```python
from build123d import *

# Parameters (mm, degrees)
BOSS_EXTRUDE1_DEPTH = 6
SKETCH3_R           = 3.5
SKETCH3_R_2         = 7
CUT_EXTRUDE1_DEPTH  = 83.160412203
FILLET1_R           = 2


with BuildPart() as part:
    # Sketch1 → Revolve1 (revolve)
    with BuildSketch(Plane(origin=(0, 0, 0), x_dir=(0, 0, -1), z_dir=(1, 0, 0)), mode=Mode.PRIVATE) as revolve1_sk:
        with BuildLine():
            Line((-3, 45), (-3, 26))
            ThreePointArc((-3, 26), (-3.878679656, 23.878679656), (-6, 23))
            Line((-6, 23), (-7, 23))
            Line((-7, 23), (-7, 7))
            Line((-7, 7), (0, 7))
            Line((0, 7), (0, 19))
            Line((0, 19), (8, 19))
            Line((8, 19), (8, 40))
            Line((8, 40), (14, 40))
            Line((14, 40), (14, 45))
            Line((14, 45), (3, 45))
            Line((3, 45), (-3, 45))
        make_face()
    revolve(revolve1_sk.sketch.rotate(Axis((0, 0, 21.063158719), (0, 0, -1)), 90), axis=Axis((0, 0, 21.063158719), (0, 0, -1)))

    # Sketch2 → Boss-Extrude1 (add)
    with BuildSketch(Plane.XY):
        Polygon((0, 61.199128534), (-53, 30.599564267), (-53, -30.599564267), (0, -61.199128534), (53, -30.599564267), (53, 30.599564267), align=None)
    extrude(amount=-BOSS_EXTRUDE1_DEPTH)

    # Sketch3 → Cut-Extrude1 (cut, through all)
    with BuildSketch(Plane.XY):
        with Locations((0, 51)):
            Circle(SKETCH3_R)
        with Locations((44.167295593, 25.5)):
            Circle(SKETCH3_R)
        with Locations((44.167295593, -25.5)):
            Circle(SKETCH3_R)
        with Locations((0, -51)):
            Circle(SKETCH3_R)
        with Locations((-44.167295593, -25.5)):
            Circle(SKETCH3_R)
        with Locations((-44.167295593, 25.5)):
            Circle(SKETCH3_R)
        Circle(SKETCH3_R_2)
    extrude(amount=-CUT_EXTRUDE1_DEPTH, mode=Mode.SUBTRACT)

    # Fillet1
    fillet1_edges = [part.edges().sort_by_distance(p)[0] for p in [
        (26.5, 45.899346401, 0),
        (-26.5, 45.899346401, 0),
        (-53, 0, 0),
        (-26.5, -45.899346401, 0),
        (26.5, -45.899346401, 0),
        (53, 0, 0),
    ]]
    fillet(fillet1_edges, radius=FILLET1_R)


solid = part.part
```
Source: CAD feature listing. Evaluate the final solid. Frame: model axes, mm. A direction names the side the tool comes from. Round coordinates to 2 decimals unless told otherwise and drop trailing zeros.
(1) Access query for faces 1 (the cylindrical face through (-4.119, 18.548, -7.014)), 2 (the flat face through (-26.129, 46.114, -3.972)), 3 (the cylindrical face through (-2.994, -22.804, 6.507)). Directions: +Z, -Z, +X, -X, +Y, -Y. A direction counts if a zero-diameter tool reaches every point of the face in a straight line with its end or side. Return the directions, or none.
From the geometry:
face 1: -Z
face 2: +Z, -Z, -X, +Y
face 3: +Z
(2) Material intervals for probe 1 along Y at (x, z) = (0, -4.35); probe 2 along Y at (x, z) = (0, -6.95); probe 3 along Y at (x, z) = (0, 0.75), sorted ascending.
From the geometry:
probe 1: y = -61.2 to -54.5, -47.5 to -7, 7 to 47.5, 54.5 to 61.2
probe 2: y = -45 to -19, 19 to 45
probe 3: y = -45 to -7, 7 to 45
(3) Pull-direction query (X, two-part tool) for faces 4 (the cylindrical face through (25.83, 45.59, -0.57)), 5 (the cylindrical face through (3.23, 6.21, 0.41)), 6 (the cylindrical face through (20.765, 39.923, 1.521)), 7 (the flat face through (19, 19, 3)); classes: +X half, -X half, draft (parallel to the pull), parting line (faces both ways), or undercut.
From the geometry:
face 4: +X half
face 5: undercut
face 6: parting line
face 7: draft
(4) Contact query for flat-ended pins moving along their axis: pin 1 Ø6.5 at (x, y) = (44.17, 25.5) entering from +Z; pin 2 Ø19 at (x, y) = (-8.5, -3) entering from -Z; pin 3 Ø1 at (x, z) = (-23.5, -7) entering from +Y; pin 4 Ø5 at (x, z) = (41, -9.5) entering from +Y. Output: stop coordinate, or through.
From the geometry:
pin 1: passes through
pin 2: stops at z = -6
pin 3: stops at y = 38.68
pin 4: stops at y = 23.3
